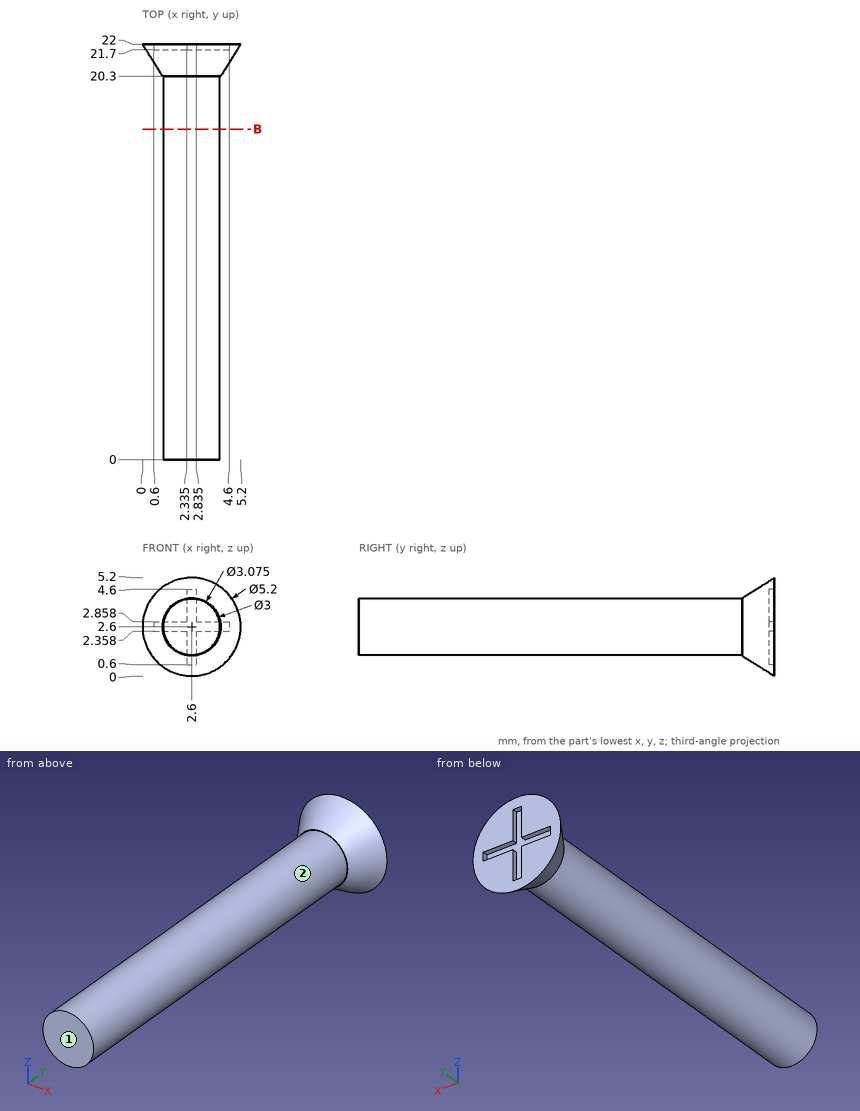
Could you check a few things on this drawing? It's one solid part, dimensions in mm from its lowest x, y, z. A direction names the side the tool comes from. Coordinates: 2 decimals unless noted, no trailing zeros. Write each loop counter-clockwise with the first axis right and the second up, starting at its lowest first coordinate (ties: lowest second). Pieces come first, ordered by that corner, then holes. Notation, with made-up numbers: (22.25, 33.25) - (72.25, 33.25) arc R32 cw to (72.25, 63.25) - close; hole circle Ø1 at (0, 15.25). An arc over 180 degrees is marked (long way). Return JSON: item names as keys, results as strings. Group by question number.
Item 1: Please list where these lines run through material, in increasing order: probe 1 along Y at (x, z) = (3, 4.2) (1 decimal); probe 2 along X at (y, z) = (11.25, 2.1) (1 decimal); probe 3 along Z at (x, y) = (1.6, 14.25).
Item 2: If we section it at B-B (y = 17.5): Write out the boundary of the cut face in (x, z).
Item 3: Which directions (+Z, -Z, +X, -X, +Y, -Y) give clear straight access to the entire face, cutting with the end or side of a thin tool? Please do the marked faces 1 and 2.
Item 4: I'm going to push flat-ended pins straight in: pin 1 Ø3 at (x, y) = (1, 17) entering from +Z; pin 2 Ø1 at (y, z) = (12, 3) entering from -X; pin 3 Ø1 at (y, z) = (15.5, 1) entering from +X. Where does each tip first touch, or does it pass through?
Return value:
{
 "1": {"probe 1": "y = 20.5 to 22", "probe 2": "x = 1.2 to 4", "probe 3": "z = 1.48 to 3.72"},
 "2": {"outline": "circle Ø3 at (2.6, 2.6)"},
 "3": {"face 1": "+Z, -Z, +X, -X, -Y", "face 2": "-Y"},
 "4": {"pin 1": "stops at z = 4.1", "pin 2": "stops at x = 1.1", "pin 3": "stops at x = 3.62"}
}
